```python
from build123d import *

# Parameters (mm, degrees)
F0_R     = 9.525
F1_DEPTH = 6.35


with BuildPart() as f1:
    # F0 (on Front) → F1 (new body)
    with BuildSketch(Plane.XZ):
        with BuildLine():
            ThreePointArc((15.747944, -2.004468), (10.943676, 1.929665), (14.112658, 7.269697))
            ThreePointArc((14.112658, 7.269697), (13.748153, 7.9375), (13.352072, 8.587072))
            ThreePointArc((13.352072, 8.587072), (7.142977, 8.512669), (6.138052, 14.640353))
            ThreePointArc((6.138052, 14.640353), (5.42957, 14.91762), (4.708617, 15.160625))
            ThreePointArc((4.708617, 15.160625), (0, 11.1125), (-4.708617, 15.160625))
            ThreePointArc((-4.708617, 15.160625), (-5.42957, 14.91762), (-6.138052, 14.640353))
            ThreePointArc((-6.138052, 14.640353), (-5.619131, 13.448613), (-5.441753, 12.160956))
            ThreePointArc((-5.441753, 12.160956), (-8.243396, 7.820858), (-13.352072, 8.587072))
            ThreePointArc((-13.352072, 8.587072), (-13.748153, 7.9375), (-14.112658, 7.269697))
            ThreePointArc((-14.112658, 7.269697), (-11.765622, 5.534871), (-10.871323, 2.756665))
            ThreePointArc((-10.871323, 2.756665), (-12.306819, -0.65104), (-15.747944, -2.004468))
            ThreePointArc((-15.747944, -2.004468), (-15.633823, -2.756665), (-15.483795, -3.502531))
            ThreePointArc((-15.483795, -3.502531), (-11.063436, -4.003838), (-8.985653, -7.9375))
            ThreePointArc((-8.985653, -7.9375), (-9.456289, -10.001793), (-10.775178, -11.658094))
            ThreePointArc((-10.775178, -11.658094), (-10.204253, -12.160956), (-9.609892, -12.635886))
            ThreePointArc((-9.609892, -12.635886), (-4.252153, -10.302959), (-0.66707, -14.91762))
            ThreePointArc((-0.66707, -14.91762), (-0.690507, -15.389517), (-0.760586, -15.856769))
            ThreePointArc((-0.760586, -15.856769), (0, -15.875), (0.760586, -15.856769))
            ThreePointArc((0.760586, -15.856769), (3.800699, -10.442334), (9.609892, -12.635886))
            ThreePointArc((9.609892, -12.635886), (10.204253, -12.160956), (10.775178, -11.658094))
            ThreePointArc((10.775178, -11.658094), (9.623707, -5.55625), (15.483795, -3.502531))
            ThreePointArc((15.483795, -3.502531), (15.633823, -2.756665), (15.747944, -2.004468))
        make_face()
        Circle(F0_R, mode=Mode.SUBTRACT)
    extrude(amount=F1_DEPTH)


solid = f1.part
```
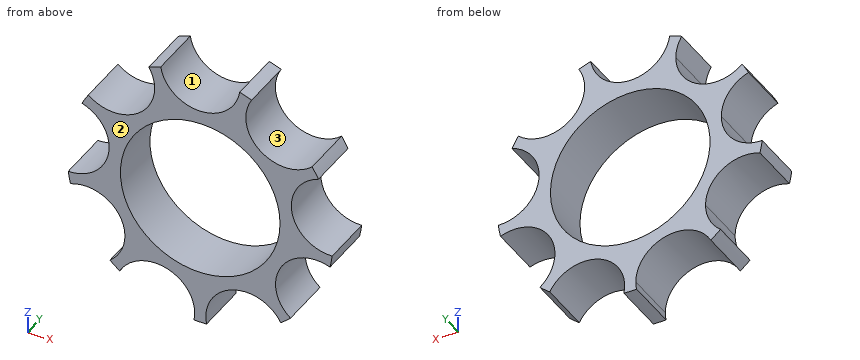
Input: part model. Units: mm. Frame: model coordinates. Face numbers are marked on the shaded views. Give positions to 0.01 mm unless a question says otherwise; leave off trailing zeros. Write each loop counter-clockwise with the first axis right and the second up, starting at its lowest first coordinate (ties: lowest second). Pieces come first, ordered by that corner, then holes. Notation, with made-up numbers: (20, 22) - (61, 22) arc R10 cw to (61, 38) - close; hole circle Ø4 at (2, 66). An arc over 180 degrees is marked (long way). Write item = value, one per line. Start each with the question number.
1) Cut plane C-C (z = 2). Return loops of the section in (x, y), and give its area (3 significant figures).
2) Material intervals for L1, parallel to X at y = -4, z = -11.5; L2, parallel to X at y = -3, z = -12; L3, parallel to X at y = -2.75, z = -14, sorted ascending. Write a range as [from, to].
3) Cut plane D-D (z = -13). Return loops of the section in (x, y).
4) Draft query along Z for the marked faces 1, 2 and 3. Return one class per face: pulls with the +Z half, pulls with the -Z half, needs draft (parallel to the pull), parting line crosses it, or undercut.
5) Pin query (flat end, axial travel): pin 1 (15 mm diameter, centred on x = 0, z = 0, fed in from +Y); pin 2 (1 mm diameter, centred on x = 7, y = -2, fed in from -Z); pin 3 (3 mm diameter, centred on x = 9, y = -4.5, fed in from -Z); pin 4 (1 mm diameter, centred on x = -1, y = -2, fed in from +Z). Return the tip coordinate at first contact, or that it passes through.
Answers follow:
q1.outline = (-10.93, -6.35) - (-9.31, -6.35) - (-9.31, 0) - (-10.93, 0) - close; (9.31, -6.35) - (10.93, -6.35) - (10.93, 0) - (9.31, 0) - close
q1.area = 20.6 mm^2
q2.L1 = [-10.59, -8.75], [-2.11, 2.11], [8.75, 10.59]
q2.L2 = [-10.39, -9.19], [-1.67, 1.67], [9.19, 10.39]
q2.L3 = [-0.76, 0.76]
q3.outline = (-1.07, -6.35) - (1.07, -6.35) - (1.07, 0) - (-1.07, 0) - close
q4.face_1 = pulls with the +Z half
q4.face_2 = needs draft
q4.face_3 = undercut
q5.pin_1 = through
q5.pin_2 = -10.63
q5.pin_3 = -12.64
q5.pin_4 = 11.35
